```python
from build123d import *

# Parameters (mm, degrees)
SKETCH1_W           = 126
SKETCH1_H           = 126
BOSS_EXTRUDE1_DEPTH = 5
SKETCH4_W           = 76
SKETCH4_H           = 21.5
CUT_EXTRUDE3_DEPTH  = 10
CUT_EXTRUDE4_START  = -5
CUT_EXTRUDE4_DEPTH  = 5
SKETCH11_W          = 15
SKETCH11_H          = 13
BOSS_EXTRUDE2_DEPTH = 3
SKETCH12_R          = 2.95
CUT_EXTRUDE5_DEPTH  = 3
LPATTERN1_COUNT     = 2
LPATTERN1_PITCH     = 20
LPATTERN2_COUNT     = 2
LPATTERN2_PITCH     = 20
SKETCH13_W          = 51
SKETCH13_H          = 34.5
CUT_EXTRUDE6_DEPTH  = 179.370401132
SKETCH14_W          = 51
SKETCH14_H          = 34.5
CUT_EXTRUDE7_DEPTH  = 179.370401132
SKETCH17_R          = 2.95
CUT_EXTRUDE10_DEPTH = 179.370401132
SKETCH18_R          = 21.778665512
SKETCH18_R_2        = 19.5
BOSS_EXTRUDE3_DEPTH = 6
SKETCH19_W          = 44.860431558
SKETCH19_H          = 6
SKETCH19_W_2        = 6
SKETCH19_H_2        = 44.549983506
CUT_EXTRUDE11_DEPTH = 6
SKETCH21_R          = 15.75
CUT_EXTRUDE14_DEPTH = 179.530109505
CUT_EXTRUDE15_DEPTH = 2.5


# Read off the part's stored shape, not the designer's step: Cut-Extrude4
with BuildPart() as part:
    # Sketch1 → Boss-Extrude1 (new body)
    with BuildSketch(Plane(origin=(0, 0, 0), x_dir=(1, 0, 0), z_dir=(0, 1, 0))):
        with Locations((63, 63)):
            Rectangle(SKETCH1_W, SKETCH1_H)
    extrude(amount=BOSS_EXTRUDE1_DEPTH)

    # Sketch4 → Cut-Extrude3 (cut)
    with BuildSketch(Plane(origin=(0, 5, 0), x_dir=(1, 0, 0), z_dir=(0, 1, 0))):
        with Locations((81.213909597, 22.875)):
            Rectangle(SKETCH4_W, SKETCH4_H)
    extrude(amount=-CUT_EXTRUDE3_DEPTH, mode=Mode.SUBTRACT)

    # Cut-Extrude4 outline → Cut-Extrude4 (cut)
    with BuildSketch(Plane(origin=(0, 5, 0), x_dir=(1, 0, 0), z_dir=(0, 1, 0)).offset(CUT_EXTRUDE4_START)):
        Polygon((46.623568796, 109.033538796), (51.912030335, 103.132096488), (46.436068796, 97.033538796), (50.116357258, 97.033538796), (53.750972642, 101.079211873), (57.375972642, 97.033538796), (61.051453412, 97.033538796), (55.58991495, 103.129692642), (60.892799565, 109.033538796), (57.210107258, 109.033538796), (53.750972642, 105.180173411), (50.299049565, 109.033538796), align=None)
        Polygon((26.586259271, 109.023073742), (31.87472081, 103.121631435), (26.398759271, 97.023073742), (30.079047733, 97.023073742), (33.713663117, 101.068746819), (37.338663117, 97.023073742), (41.014143886, 97.023073742), (35.552605425, 103.119227588), (40.85549004, 109.023073742), (37.172797733, 109.023073742), (33.713663117, 105.169708358), (30.26174004, 109.023073742), align=None)
    extrude(amount=CUT_EXTRUDE4_DEPTH, mode=Mode.SUBTRACT)

    # Sketch11 → Boss-Extrude2 (add)
    with BuildSketch(Plane.XZ):
        with Locations((53.750972642, -103.129692642)):
            Rectangle(SKETCH11_W, SKETCH11_H)
    boss_extrude2 = extrude(amount=BOSS_EXTRUDE2_DEPTH)

    # Sketch12 → Cut-Extrude5 (cut)
    with BuildSketch(Plane.XZ.offset(3)):
        with Locations(Location((53.750972642, -103.129692642, 0), (0, 0, 270))):
            Circle(SKETCH12_R)
    cut_extrude5 = extrude(amount=-CUT_EXTRUDE5_DEPTH, mode=Mode.SUBTRACT)

    # LPattern1: Boss-Extrude2 ×2
    with Locations(*[(-i * LPATTERN1_PITCH, 0, 0) for i in range(1, LPATTERN1_COUNT)]):
        add(boss_extrude2)

    # LPattern2: Cut-Extrude5 ×2
    with Locations(*[(-i * LPATTERN2_PITCH, 0, 0) for i in range(1, LPATTERN2_COUNT)]):
        add(cut_extrude5, mode=Mode.SUBTRACT)

    # Sketch13 → Cut-Extrude6 (cut, through all)
    with BuildSketch(Plane(origin=(0, 5, 0), x_dir=(1, 0, 0), z_dir=(0, 1, 0))):
        with Locations((32.5, 63)):
            Rectangle(SKETCH13_W, SKETCH13_H)
    extrude(amount=-CUT_EXTRUDE6_DEPTH, mode=Mode.SUBTRACT)

    # Sketch14 → Cut-Extrude7 (cut, through all)
    with BuildSketch(Plane(origin=(0, 5, 0), x_dir=(1, 0, 0), z_dir=(0, 1, 0))):
        with Locations((93.5, 63)):
            Rectangle(SKETCH14_W, SKETCH14_H)
    extrude(amount=-CUT_EXTRUDE7_DEPTH, mode=Mode.SUBTRACT)

    # Sketch17 → Cut-Extrude10 (cut, through all)
    with BuildSketch(Plane(origin=(0, 5, 0), x_dir=(1, 0, 0), z_dir=(0, 1, 0))):
        with Locations(Location((63, 55.625, 0), (0, 0, 270))):
            Circle(SKETCH17_R)
        with Locations(Location((63, 70.940065171, 0), (0, 0, 270))):
            Circle(SKETCH17_R)
    extrude(amount=-CUT_EXTRUDE10_DEPTH, mode=Mode.SUBTRACT)

    # Sketch18 → Boss-Extrude3 (add)
    with BuildSketch(Plane.XZ):
        with Locations(Location((93.5, -103.125, 0), (0, 0, 270))):
            Circle(SKETCH18_R)
        with Locations(Location((93.5, -103.125, 0), (0, 0, 270))):
            Circle(SKETCH18_R_2, mode=Mode.SUBTRACT)
    extrude(amount=BOSS_EXTRUDE3_DEPTH)

    # Sketch19 → Cut-Extrude11 (cut)
    with BuildSketch(Plane.XZ.offset(6)):
        with Locations((93.5, -103.125)):
            Rectangle(SKETCH19_W, SKETCH19_H)
        with Locations((93.5, -103.125)):
            Rectangle(SKETCH19_W_2, SKETCH19_H_2)
    extrude(amount=-CUT_EXTRUDE11_DEPTH, mode=Mode.SUBTRACT)

    # Sketch21 → Cut-Extrude14 (cut, through all)
    with BuildSketch(Plane(origin=(0, 5, 0), x_dir=(1, 0, 0), z_dir=(0, 1, 0))):
        with Locations(Location((93.5, 103.125, 0), (0, 0, 270))):
            Circle(SKETCH21_R)
    extrude(amount=-CUT_EXTRUDE14_DEPTH, mode=Mode.SUBTRACT)

    # Sketch22 → Cut-Extrude15 (cut)
    with BuildSketch(Plane(origin=(0, 5, 0), x_dir=(1, 0, 0), z_dir=(0, 1, 0))):
        with BuildLine():
            ThreePointArc((78.650757595, 97.875), (77.75, 103.125), (78.650757595, 108.375))
            Line((78.650757595, 108.375), (76.75, 108.375))
            Line((76.75, 108.375), (76.75, 97.875))
            Line((76.75, 97.875), (78.650757595, 97.875))
        make_face()
        with BuildLine():
            ThreePointArc((88.25, 117.974242405), (93.5, 118.875), (98.75, 117.974242405))
            Line((98.75, 117.974242405), (98.75, 119.875))
            Line((98.75, 119.875), (88.25, 119.875))
            Line((88.25, 119.875), (88.25, 117.974242405))
        make_face()
        with BuildLine():
            Line((110.25, 97.875), (110.25, 108.375))
            Line((110.25, 108.375), (108.349242405, 108.375))
            ThreePointArc((108.349242405, 108.375), (109.023177315, 105.788356165), (109.25, 103.125))
            ThreePointArc((109.25, 103.125), (109.023177315, 100.461643835), (108.349242405, 97.875))
            Line((108.349242405, 97.875), (110.25, 97.875))
        make_face()
        with BuildLine():
            Line((98.75, 86.375), (98.75, 88.275757595))
            ThreePointArc((98.75, 88.275757595), (93.5, 87.375), (88.25, 88.275757595))
            Line((88.25, 88.275757595), (88.25, 86.375))
            Line((88.25, 86.375), (98.75, 86.375))
        make_face()
    extrude(amount=-CUT_EXTRUDE15_DEPTH, mode=Mode.SUBTRACT)


solid = part.part
```
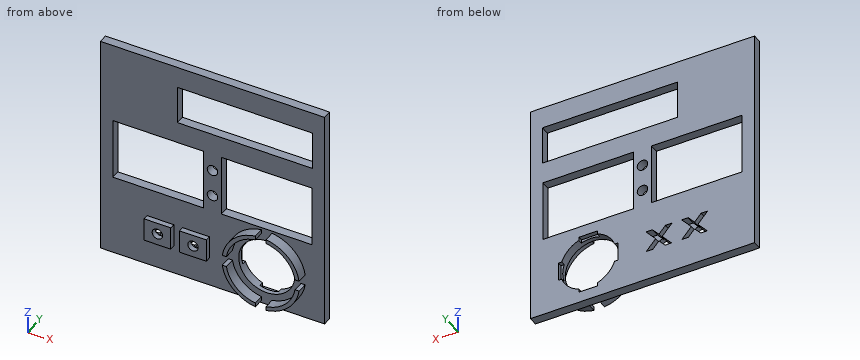
The model under review builds one solid part; all positions refer to its coordinate system, in mm. Give positions to 0.01 mm unless a question says otherwise; leave off trailing zeros. Write each loop counter-clockwise with the first axis right and the second up, starting at its lowest first coordinate (ties: lowest second). Pieces come first, ordered by that corner, then holes. Notation, with made-up numbers: (27.5, -28.75) -> (70.5, -28.75) arc R13 cw to (70.5, -16.75) -> close; hole circle Ø7 at (81, 4). An arc over 180 degrees is marked (long way). Put each result on its own line as item: value.
(1) For pin 1 Ø6 at (x, y) = (79.5, -4.5) entering from +Z; pin 2 Ø6 at (x, z) = (31.5, -47.5) entering from -Y; pin 3 Ø4 at (x, z) = (32.5, -101.5) entering from -Y, all flat-tipped, find the tip position at first contact; note any pin that passes through.
Results are:
pin 1: z = -84.33
pin 2: y = 0
pin 3: y = -3
(2) To check wall thickness, follow probe 1 along X at (y, z) = (4.5, -22); probe 2 along Z at (x, y) = (70, 2.75) (3 decimals); probe 3 along Z at (x, y) = (50, 1) (3 decimals). State the ranges of each line that lie inside material, in increasing order. Write a range as from..to.
Results are:
probe 1: 0..43.21, 119.21..126
probe 2: -126..-80.25, -45.75..-33.625, -12.125..0
probe 3: -126..-109.034, -105.266..-101.003, -97.034..-80.25, -45.75..-33.625, -12.125..0
(3) We need section D-D, the plane z = -39. Give the boundary of the cut face in (x, y), and give its area (3 significant figures).
Results are:
outline: (0, 0) -> (126, 0) -> (126, 5) -> (0, 5) -> close
area: 630 mm²
(4) We need section A-A, the plane x = 63. Give the boundary of the cut face in (y, z) (3 decimals), and give its area (4 significant figures).
Results are:
outline: (0, -126) -> (5, -126) -> (5, -73.89) -> (0, -73.89) -> close; (0, -67.99) -> (5, -67.99) -> (5, -58.575) -> (0, -58.575) -> close; (0, -52.675) -> (5, -52.675) -> (5, -33.625) -> (0, -33.625) -> close; (0, -12.125) -> (5, -12.125) -> (5, 0) -> (0, 0) -> close
area: 463.5 mm²
(5) We need section C-C, the plane x = 93.5. Give the boundary of the cut face in (y, z) (3 decimals), and give its area (4 significant figures).
Results are:
outline: (0, -126) -> (5, -126) -> (5, -119.875) -> (2.5, -119.875) -> (2.5, -118.875) -> (0, -118.875) -> close; (0, -87.375) -> (2.5, -87.375) -> (2.5, -86.375) -> (5, -86.375) -> (5, -80.25) -> (0, -80.25) -> close; (0, -45.75) -> (5, -45.75) -> (5, -33.625) -> (0, -33.625) -> close; (0, -12.125) -> (5, -12.125) -> (5, 0) -> (0, 0) -> close
area: 187.5 mm²
(6) We need section B-B, the plane z = -116. Give the boundary of the cut face in (x, y).
Results are:
outline: (0, 0) -> (75.93, 0) -> (75.93, -6) -> (78.85, -6) -> (78.85, 0) -> (84.43, 0) -> (84.43, 5) -> (0, 5) -> close; (102.57, 0) -> (108.15, 0) -> (108.15, -6) -> (111.07, -6) -> (111.07, 0) -> (126, 0) -> (126, 5) -> (102.57, 5) -> close
